Could you check a few things on this model? Use its own coordinates, in mm. Face numbers are marked on the shaded views. A direction names the side the tool comes from. Round coordinates to 2 decimals unless told otherwise and drop trailing zeros. Write each loop counter-clockwise with the first axis right and the second up, starting at its lowest first coordinate (ties: lowest second). Pieces come first, ordered by that corner, then holes. Notation, with made-up numbers: (5, 80) -> (17, 80) arc R6 ccw to (17, 87) -> close; hole circle Ø8 at (3.5, 20). An arc over 180 degrees is marked (long way). One line per question, with ' | ' between items. Start each with the question number.
1. If I drill on line 1 along X through (y, z) = (-4.7, 0); line 2 along X through (y, z) = (4.55, 0); line 3 along Z through (x, y) = (-6, -1.75), over which ranges is the centre line in solid material (lowest first)? Write a range as [from, to].
2. Imagine slicing it at D-D, the plane x = 36. List the corners of the cut face in (y, z) for me.
3. Imagine slicing it at A-A, the plane y = 0. List the corners of the cut face in (x, z) for me, and give its area (3 significant figures).
4. Imagine slicing it at B-B, the plane x = 0. List the corners of the cut face in (y, z) for me.
5. For pin 1 Ø5 at (y, z) = (-1, -9.5) entering from +X; pin 2 Ø6 at (x, y) = (23.5, -2.5) entering from +Z; pin 3 Ø1 at (x, y) = (10, 3.5) entering from +Z, each with a flat end and sliding along its axis, tell me the tip position at first contact or that it passes through.
6. For the marked faces 1 and 2, which set-ups out of +Z, -Z, +X, -X, +Y, -Y let a thin tool reach every point of the face, with its end or its side?
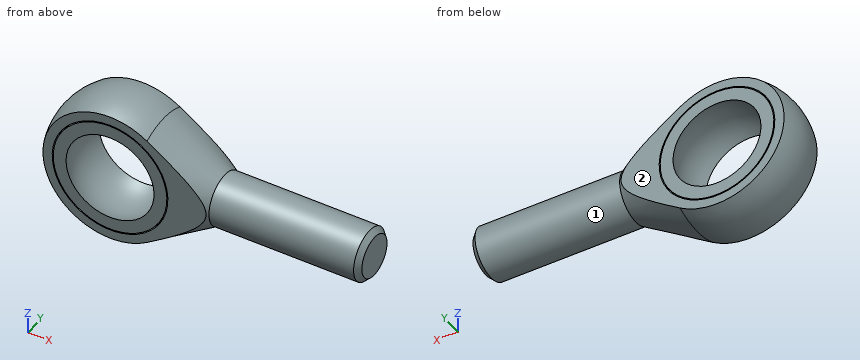
from build123d import *

# Parameters (mm, degrees)
CUT_EXTRUDE1_DEPTH      = 28.440845468
CUT_EXTRUDE1_DEPTH_BACK = 28.440845468
SKETCH3_W               = 33
SKETCH3_H               = 8.75
SKETCH4_W               = 0.2
SKETCH4_H               = 1
SKETCH5_R               = 5
BOSS_EXTRUDE1_DEPTH     = 29
CHAMFER1_SIZE           = 1


with BuildPart() as part:
    # Sketch2 → Revolve2 (revolve)
    with BuildSketch(Plane(origin=(0, 0, 0), x_dir=(1, 0, 0), z_dir=(0, 1, 0))):
        with BuildLine():
            Line((7.147970434, 12.037712352), (19, 5))
            Line((19, 5), (19, 0))
            Line((19, 0), (-14, 0))
            ThreePointArc((-14, 0), (-6.925619609, 12.166996056), (7.147970434, 12.037712352))
        make_face()
    revolve(axis=Axis((-39.456415939, 0, 0), (1, 0, 0)))

    # Sketch3 → Cut-Extrude1 (cut, two sides: drawn at the far end of the back side and taken through both)
    with BuildSketch(Plane.XY.offset(-CUT_EXTRUDE1_DEPTH_BACK)):
        with Locations((2.5, 9.625)):
            Rectangle(SKETCH3_W, SKETCH3_H)
        with Locations((2.5, -9.625)):
            Rectangle(SKETCH3_W, SKETCH3_H)
    extrude(amount=CUT_EXTRUDE1_DEPTH + CUT_EXTRUDE1_DEPTH_BACK, mode=Mode.SUBTRACT)

    # Sketch4 → Cut-Revolve1 (revolve, cut)
    with BuildSketch(Plane.XY, mode=Mode.PRIVATE) as cut_revolve1_sk:
        with BuildLine():
            Line((0, 10), (0, -10))
            ThreePointArc((0, -10), (10, 0), (0, 10))
        make_face()
        with Locations((11.1, 4.75)):
            Rectangle(SKETCH4_W, SKETCH4_H)
        with Locations((11.1, -4.75)):
            Rectangle(SKETCH4_W, SKETCH4_H)
    revolve(cut_revolve1_sk.sketch.rotate(Axis((0, 13.975998128, 0), (0, -1, 0)), 90), axis=Axis((0, 13.975998128, 0), (0, -1, 0)), mode=Mode.SUBTRACT)

    # Sketch5 → Boss-Extrude1 (add)
    with BuildSketch(Plane(origin=(19, 0, 0), x_dir=(0, 0, -1), z_dir=(1, 0, 0))):
        with Locations(Location((0, 0, 0), (0, 0, 180))):
            Circle(SKETCH5_R)
    extrude(amount=BOSS_EXTRUDE1_DEPTH)

    # Chamfer1
    chamfer1_edges = [part.edges().sort_by_distance(p)[0] for p in [
        (48, 0, -5),
    ]]
    chamfer(chamfer1_edges, length=CHAMFER1_SIZE)


solid = part.part
Geometry results:
1) line 1: x = [-13.19, -11.2], [-11, -8.83], [8.83, 11], [11.2, 47.3] | line 2: x = [-13.24, -11.2], [-11, -8.9], [8.9, 11], [11.2, 47.45] | line 3: z = [-12.53, -7.81], [7.81, 12.53]
2) outline: circle Ø10 at (0, 0)
3) outline: (7.15, -12.04) -> (19, -5) -> (47, -5) -> (48, -4) -> (48, 4) -> (47, 5) -> (19, 5) -> (7.15, 12.04) arc R14 ccw (long way) to start; hole circle Ø20 at (0, 0) | area: 676 mm2
4) outline: (-5.25, -12.98) arc R14 ccw to (5.25, -12.98) -> (5.25, -11.2) -> (4.25, -11.2) -> (4.25, -11) -> (5.25, -11) -> (5.25, -8.51) arc R10 cw to (-5.25, -8.51) -> (-5.25, -11) -> (-4.25, -11) -> (-4.25, -11.2) -> (-5.25, -11.2) -> close; (-5.25, 8.51) arc R10 cw to (5.25, 8.51) -> (5.25, 11) -> (4.25, 11) -> (4.25, 11.2) -> (5.25, 11.2) -> (5.25, 12.98) arc R14 ccw to (-5.25, 12.98) -> (-5.25, 11.2) -> (-4.25, 11.2) -> (-4.25, 11) -> (-5.25, 11) -> close
5) pin 1: stops at x = 15.54 | pin 2: stops at z = 5 | pin 3: stops at z = 10.09
6) face 1: +X | face 2: +Z, -Z, +X, -X, +Y
